Here's how the part is built. I have some questions about the finished solid (model axes, mm). A direction names the side the tool comes from. Round coordinates to 2 decimals unless told otherwise and drop trailing zeros. Order: outer loops, then holes, each group sorted by start corner. A loop starts at its lowest first (then second) coordinate and runs counter-clockwise, first axis right, second up. Notation, with made-up numbers: (3, 43) -> (25, 43) arc R21 ccw to (25, 59) -> close; hole circle Ø11 at (42, 57). An arc over 180 degrees is marked (long way). Use a Markdown table: item, result. Add a question column.
(1) I'm going to push flat-ended pins straight in: P1, Ø3, axis at x = 73, y = 2.5, coming from the +Z side; P2, Ø18.5, axis at x = 107, y = 13, coming from the +Z side; P3, Ø6, axis at x = 107, z = 153, coming from the -Y side. Where does each tip first touch, or does it pass through?
(2) If I drill on probe 1 along Z at (x, y) = (100.5, 10); probe 2 along Y at (x, z) = (98, 140); probe 3 along Y at (x, z) = (92, 215), over which ranges is the centre line in solid material (lowest first)?
(3) I want a section at B-B, the plane z = 215. Please give me the cut outline in (x, y), then the cut area to 3 significant figures.
(4) I want a section at C-C, the plane y = 12.5. Please give me the cut outline in (x, z), then the cut area to 3 significant figures.
(5) I want a section at A-A, the plane x = 56.5. Please give me the cut outline in (y, z).
(6) On a 3-axis mill with a long thin cutter (end or side, diameter ignored), from which of +Z, -Z, +X, -X, +Y, -Y can I reach the whole of each face in a straight line? I mean faces 1 (the face through (88, 18, 201.3)), 2 (the face through (88, 74, 201.3)), 3 (the face through (88, 45, 0)). Say none if no direction works.
Autodesk Inventor part; units mm, degrees
ref_plane "YZ Plane" through (0, 0, 0) normal (1, 0, 0) x (0, 1, 0)
ref_plane "XZ Plane" through (0, 0, 0) normal (0, 1, 0) x (-1, 0, 0)
ref_plane "XY Plane" through (0, 0, 0) normal (0, 0, 1) x (1, 0, 0)
sketch "Sketch1" plane through (0, 0, 0) normal (0, 0, 1) x (1, 0, 0)
  line L0 (0, 0) -> (177.8, 0)
  line L1 (177.8, 0) -> (177.8, 88.9)
  line L2 (177.8, 88.9) -> (0, 88.9)
  line L3 (0, 88.9) -> (0, 0)
  dimension "d0" = 88.9
  dimension "d1" = 177.8
extrude "Extrusion1" add sketch "Sketch1" along normal blind 241.3
sketch "Sketch2" plane through (0, 0, 0) normal (0, -1, 0) x (1, 0, 0)
  line L0 (0, 0) -> (0, 241.3)
  line L1 (177.8, 0) -> (177.8, 241.3)
  line L2 (0, 203.2) -> (177.8, 203.2)
  line L3 (177.8, 203.2) -> (177.8, 127)
  line L4 (177.8, 127) -> (0, 127)
  line L5 (0, 127) -> (0, 203.2)
  line L6 (0, 0) -> (177.8, 0)
  dimension "d4" = 203.2
  dimension "d5" = 127
extrude "Extrusion2" cut sketch "Sketch2" against normal blind 6.35 contours L0 L2 L1 L4
sketch "Sketch3" plane through (0, 0, 241.3) normal (0, 0, 1) x (1, 0, 0)
  line L0 (177.8, 0) -> (177.8, 88.9)
  line L1 (0, 0) -> (177.8, 0)
  line L2 (177.8, 0) -> (177.8, 29.45)
  line L3 (177.8, 29.45) -> (0, 29.45)
  line L4 (0, 29.45) -> (0, 0)
  line L5 (0, 88.9) -> (0, 0)
  line L6 (0, 88.9) -> (177.8, 88.9)
  line L7 (177.8, 88.9) -> (177.8, 59.45)
  line L8 (177.8, 59.45) -> (0, 59.45)
  line L9 (0, 59.45) -> (0, 88.9)
  line L10 (88.9, 29.45) -> (88.9, 59.45) construction
  point P0 (0, 44.45)
  point P1 (88.9, 44.45)
  dimension "d8" = 30
extrude "Extrusion3" cut sketch "Sketch3" against normal blind 40 contours L1 L4 L3 L0 | L8 L5 L6 L0
properties part number "Battery_278Wh" material "ABS Plastic"
Taken from the geometry:
| question | item | result |
|---|---|---|
| 1 | P1 | stops at z = 127 |
| 1 | P2 | stops at z = 201.3 |
| 1 | P3 | stops at y = 6.35 |
| 2 | probe 1 | z = 0 to 201.3 |
| 2 | probe 2 | y = 6.35 to 88.9 |
| 2 | probe 3 | y = 29.45 to 59.45 |
| 3 | outline | (0, 29.45) -> (177.8, 29.45) -> (177.8, 59.45) -> (0, 59.45) -> close |
| 3 | area | 5,330 mm2 |
| 4 | outline | (0, 0) -> (177.8, 0) -> (177.8, 201.3) -> (0, 201.3) -> close |
| 4 | area | 35,800 mm2 |
| 5 | outline | (0, 0) -> (88.9, 0) -> (88.9, 201.3) -> (59.45, 201.3) -> (59.45, 241.3) -> (29.45, 241.3) -> (29.45, 201.3) -> (6.35, 201.3) -> (6.35, 127) -> (0, 127) -> close |
| 6 | face 1 | +Z, +X, -X, -Y |
| 6 | face 2 | +Z, +X, -X, +Y |
| 6 | face 3 | -Z, +X, -X, +Y, -Y |
